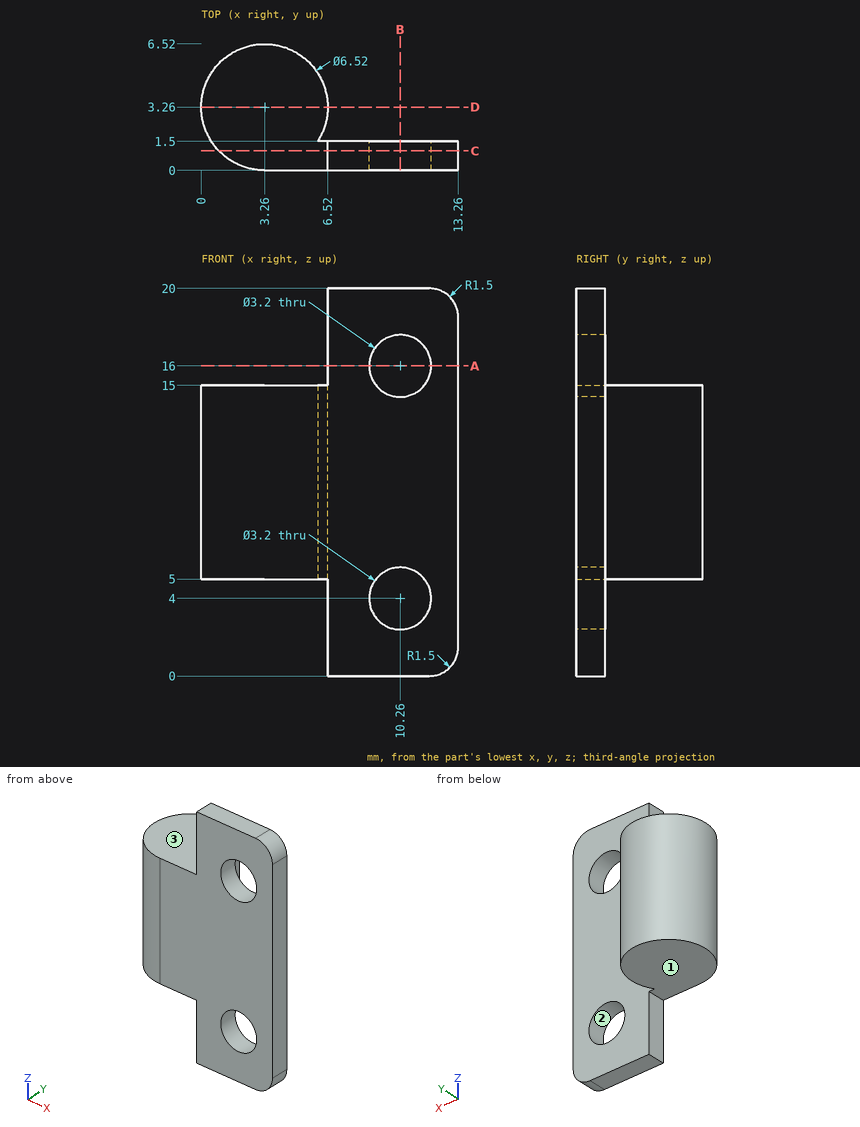
Can you work these out from the drawing? Everything is in mm from the part's minimum corner. Round coordinates to 2 decimals unless told otherwise and drop trailing zeros. Write each loop counter-clockwise with the first axis right and the second up, starting at its lowest first coordinate (ties: lowest second). Pieces come first, ordered by that corner, then holes. Notation, with made-up numbers: (-1.75, 19) - (42.25, 19) arc R23 cw to (42.25, 57) - close; hole circle Ø4 at (63, 36.25). An arc over 180 degrees is marked (long way). Write each question's results on one line, items separated by ' | '. Start each with the question number.
1) For pin 1 Ø1.6 at (y, z) = (1, 2) entering from -X; pin 2 Ø2 at (x, y) = (4, 3.5) entering from -Z; pin 3 Ø3.5 at (x, z) = (11.5, 12) entering from +Y, each with a flat end and sliding along its axis, tell me the tip position at first contact or that it passes through.
2) Suppose I cut it at B-B (x = 10.26). List the corners of the cut face in (y, z) for me, and give its area (3 significant figures).
3) Please list where these lines run through material, in increasing order: line 1 (Z direction, x = 10.26, y = 1.1); line 2 (X direction, y = 0.8, z = 4); line 3 (Y direction, x = 12.5, z = 5.5).
4) Suppose I cut it at C-C (y = 1). List the corners of the cut face in (x, z) for me, and give its area (3 significant figures).
5) Suppose I cut it at D-D (y = 3.26). List the corners of the cut face in (x, z) for me.
6) We'd pull the mould along Z, two halves only. Please class the marked faces 1, 2 and 3: released by +Z, released by -Z, zero draft, split by the parting line, or undercut.
7) Suppose I cut it at A-A (z = 16). List the corners of the cut face in (x, y) for me, and give its area (3 significant figures).
Here are the results:
1) pin 1: stops at x = 6.52 | pin 2: stops at z = 5 | pin 3: stops at y = 1.5
2) outline: (0, 0) - (1.5, 0) - (1.5, 2.4) - (0, 2.4) - close; (0, 5.6) - (1.5, 5.6) - (1.5, 14.4) - (0, 14.4) - close; (0, 17.6) - (1.5, 17.6) - (1.5, 20) - (0, 20) - close | area: 20.4 mm2
3) line 1: z = 0 to 2.4, 5.6 to 14.4, 17.6 to 20 | line 2: x = 6.52 to 8.66, 11.86 to 13.26 | line 3: y = 0 to 1.5
4) outline: (0.91, 5) - (6.52, 5) - (6.52, 0) - (11.76, 0) arc R1.5 ccw to (13.26, 1.5) - (13.26, 18.5) arc R1.5 ccw to (11.76, 20) - (6.52, 20) - (6.52, 15) - (0.91, 15) - close; hole circle Ø3.2 at (10.26, 4); hole circle Ø3.2 at (10.26, 16) | area: 174 mm2
5) outline: (0, 5) - (6.52, 5) - (6.52, 15) - (0, 15) - close
6) face 1: released by -Z | face 2: undercut | face 3: released by +Z
7) outline: (6.52, 0) - (8.66, 0) - (8.66, 1.5) - (6.52, 1.5) - close; (11.86, 0) - (13.26, 0) - (13.26, 1.5) - (11.86, 1.5) - close | area: 5.31 mm2
